```python
from build123d import *


with BuildPart() as part:
    # Sketch1 → Revolve1 (revolve)
    with BuildSketch(Plane.XY):
        with BuildLine():
            Line((-6, 0), (0, 0))
            Line((0, 0), (0, 320.752985543))
            ThreePointArc((0, 320.752985543), (-8.074390693, 317.189292472), (-6.242921278, 308.555555556))
            ThreePointArc((-6.242921278, 308.555555556), (-5.614381917, 306.333333333), (-7.5, 305))
            Line((-7.5, 305), (-7.5, 19.5))
            ThreePointArc((-7.5, 19.5), (-7.939339828, 18.439339828), (-9, 18))
            Line((-9, 18), (-9, 15))
            Line((-9, 15), (-6, 15))
            Line((-6, 15), (-6, 0))
        make_face()
    revolve(axis=Axis((0, 0, 0), (0, 1, 0)))


solid = part.part
```
The listing builds one solid part. Answer for the finished solid, in the listing's coordinates (mm). A direction names the side the tool comes from. Round coordinates to 2 decimals unless told otherwise and drop trailing zeros. Loops run counter-clockwise (first coordinate to the right, second up) from the corner with the lowest first, then second, coordinate; pieces in that order, holes last.
1) Given P1, Ø6, axis at x = -6.5, z = 6.5, coming from the -Y side; P2, Ø5, axis at x = 4, y = 109, coming from the -Z side; P3, Ø3, axis at y = 162, z = 4, coming from the +X side, each flat-ended and moving along its own axis, determine where each tip first touches the part or whether it passes through.
Outcome:
P1: stops at y = 15
P2: stops at z = -7.35
P3: stops at x = 7.07
2) A cutting plane is placed at A-A on y = 290. Determine the outline of the cut face in (x, z).
Outcome:
outline: circle Ø15 at (0, 0)
3) Consider line 1 (Z direction, x = -0.25, y = 255.5); line 2 (Y direction, x = 2.25, z = -0.5); line 3 (Y direction, x = -7, z = 5.5). Determine where each line is inside the solid, lowest interval first.
Outcome:
line 1: z = -7.5 to 7.5
line 2: y = 0 to 320.98
line 3: y = 15 to 18
4) For faces 1 (the face through (0, 0, 0)), 2 (the face through (-2, 15, -6)), 3 (the face through (7.493, 160.252, 0.33)), determine the directions among +Z, -Z, +X, -X, +Y, -Y from which every point of the face is accessible in a straight line to the end or side of a thin tool.
Outcome:
face 1: +Z, -Z, +X, -X, -Y
face 2: -Y
face 3: none
